from build123d import *

# Parameters (mm, degrees)
F0_W     = 30
F0_H     = 50
F0_R     = 11.001
F1_DEPTH = 7
F2_R     = 7
F3_SIZE  = 2


with BuildPart() as f1:
    # F0 (on Top) → F1 (new body)
    with BuildSketch(Plane.XY):
        Rectangle(F0_W, F0_H)
        Circle(F0_R, mode=Mode.SUBTRACT)
    extrude(amount=F1_DEPTH)

    # F2
    f2_edges = [f1.edges().sort_by_distance(p)[0] for p in [
        (-15, -25, 3.5),
        (15, -25, 3.5),
        (-15, 25, 3.5),
        (15, 25, 3.5),
    ]]
    fillet(f2_edges, radius=F2_R)

    # F3
    f3_edges = [f1.edges().sort_by_distance(p)[0] for p in [
        (-15, 0, 7),
        (-15, 0, 0),
    ]]
    chamfer(f3_edges, length=F3_SIZE)


solid = f1.part
Build history of the part. All positions in model axes, mm. Give positions to 0.01 mm unless a question says otherwise; leave off trailing zeros. Write each loop counter-clockwise with the first axis right and the second up, starting at its lowest first coordinate (ties: lowest second). Pieces come first, ordered by that corner, then holes. Notation, with made-up numbers: (43.25, 6) - (70.25, 6) arc R22 cw to (70.25, 18) - close; hole circle Ø2 at (70, 6.25). An arc over 180 degrees is marked (long way). Use one line per item in the form item = value. Start each with the question number.
1. Band-saw the part on A-A on z = 2.5. Write the cut outline in (x, y), plus the area to 3 significant figures.
2. Two-plate mould, pull along Y, no slides. Class faces 1 (the face through (12.9, 23, 3.5)), 2 (the face through (0, -24, 6)), 3 (the face through (10.493, 3.304, 3.451)): released by +Y, released by -Y, zero draft, split by the parting line, or undercut.
3. Band-saw the part on C-C on y = 0. Write the cut outline in (x, z).
4. Probe line 1 (Y direction, x = 0, z = 4.75); line 2 (Y direction, x = 7, z = 5.5); line 3 (X direction, y = -10, z = 4.5). List the from-to ranges inside material, lowest first. Write a range as [from, to].
5. Band-saw the part on D-D on y = -14. Write the cut outline in (x, z), plus the area to 3 significant figures.
6. Band-saw the part on B-B on x = 0. Write the cut outline in (y, z), plus the area to 3 significant figures.
Conclusion:
q1.outline = (-15, -18) arc R7 ccw to (-8, -25) - (8, -25) arc R7 ccw to (15, -18) - (15, 18) arc R7 ccw to (8, 25) - (-8, 25) arc R7 ccw to (-15, 18) - close; hole circle Ø22 at (0, 0)
q1.area = 1,080 mm²
q2.face_1 = released by +Y
q2.face_2 = released by -Y
q2.face_3 = undercut
q3.outline = (-15, 2) - (-13, 0) - (-11, 0) - (-11, 7) - (-13, 7) - (-15, 5) - close; (11, 0) - (13, 0) - (15, 2) - (15, 5) - (13, 7) - (11, 7) - close
q4.line_1 = [-25, -11], [11, 25]
q4.line_2 = [-24.5, -8.49], [8.49, 24.5]
q4.line_3 = [-15, -4.58], [4.58, 15]
q5.outline = (-15, 2) - (-13, 0) - (13, 0) - (15, 2) - (15, 5) - (13, 7) - (-13, 7) - (-15, 5) - close
q5.area = 202 mm²
q6.outline = (-25, 2) - (-23, 0) - (-11, 0) - (-11, 7) - (-23, 7) - (-25, 5) - close; (11, 0) - (23, 0) - (25, 2) - (25, 5) - (23, 7) - (11, 7) - close
q6.area = 188 mm²
